Autodesk Inventor part; units mm, degrees
ref_plane "YZ Plane" through (0, 0, 0) normal (1, 0, 0) x (0, 1, 0)
ref_plane "XZ Plane" through (0, 0, 0) normal (0, 1, 0) x (-1, 0, 0)
ref_plane "XY Plane" through (0, 0, 0) normal (0, 0, 1) x (1, 0, 0)
sketch "Sketch1" plane through (0, 0, 0) normal (0, 1, 0) x (-1, 0, 0)
  line L0 (-50, 86.6025) -> (-100, 0)
  line L1 (-100, 0) -> (-50, -86.6025)
  line L2 (-50, -86.6025) -> (50, -86.6025)
  line L3 (50, -86.6025) -> (100, 0)
  line L4 (100, 0) -> (50, 86.6025)
  line L5 (50, 86.6025) -> (-50, 86.6025)
  circle A0 centre (20, -80.1075) radius 1.6
  circle A1 centre (-20, -80.1075) radius 1.6
  line L6 (-80, 0) -> (-40, 69.282)
  line L7 (-40, 69.282) -> (-20, 69.282)
  line L8 (-80, 0) -> (-40, -69.282)
  line L9 (-40, -69.282) -> (-20, -69.282)
  line L10 (20, -69.282) -> (40, -69.282)
  line L11 (40, -69.282) -> (80, 0)
  line L12 (80, 0) -> (40, 69.282)
  line L13 (40, 69.282) -> (20, 69.282)
  line L14 (-20, 69.282) -> (-20, 34.641)
  line L15 (20, 69.282) -> (20, 34.641)
  line L16 (20, -69.282) -> (20, -34.641)
  line L17 (-20, -69.282) -> (-20, -34.641)
  line L18 (-20, -34.641) -> (-40, 0)
  line L19 (-40, 0) -> (-20, 34.641)
  line L20 (20, 34.641) -> (40, 0)
  line L21 (40, 0) -> (20, -34.641)
  circle A2 centre (-10, -51.9615) radius 6.25
  circle A3 centre (10, -51.9615) radius 6.25
  circle A4 centre (-10.5, 51.9615) radius 1.65
  circle A5 centre (10.5, 51.9615) radius 1.6
  circle A6 centre (-59.3781, 57.3685) radius 1.6
  circle A7 centre (-81.8748, -18.4029) radius 1.6
  circle A8 centre (59.3781, 57.3685) radius 1.6
  circle A9 centre (81.8767, -18.3996) radius 1.6
  circle A10 centre (-30, -80.1075) radius 3
  circle A11 centre (30, -80.1075) radius 3
  dimension "d12" = 6
  dimension "d13" = 6
extrude "Extrusion1" add sketch "Sketch1" along normal blind 3
sketch "Sketch6" plane through (0, 3, 0) normal (0, 1, 0) x (1, 0, 0)
  line L0 (0, 0) -> (0, -34.641)
  line L1 (0, 0) -> (-40, 0)
  line L2 (17.5, -17.5) -> (-17.5, -17.5) construction
  line L3 (-17.5, -17.5) -> (-17.5, 17.5) construction
  line L4 (-17.5, 17.5) -> (17.5, 17.5) construction
  line L5 (17.5, 17.5) -> (17.5, -17.5) construction
  dimension "d58" = 35
  dimension "d70" = 17.5
  dimension "d72" = 17.5
decal "Decal1"
properties part number "Top Plate" material "Polycarbonate, Clear"
Can you work these out from the model? Positions are in its coordinate system, mm. A direction names the side the tool comes from. Coordinates: 2 decimals unless noted, no trailing zeros. Loops run counter-clockwise (first coordinate to the right, second up) from the corner with the lowest first, then second, coordinate; pieces in that order, holes last.
Item 1: I'm going to push flat-ended pins straight in: pin 1 (1.5 mm diameter, centred on y = 2, z = 13, fed in from +X); pin 2 (0.9 mm diameter, centred on y = 1.5, z = 50.5, fed in from -X). Where does each tip first touch, or does it pass through?
Answers below:
pin 1: stops at x = 92.93
pin 2: stops at x = -71.1
Item 2: Which directions (+Z, -Z, +X, -X, +Y, -Y) give clear straight access to the entire face, cutting with the end or side of a thin tool? Please do faces 1 (the face through (74.65, 1.48, 43.91)), 2 (the face through (60.28, 1.48, -34.16)).
Answers below:
face 1: +Z, +X, +Y, -Y
face 2: +Y, -Y
Item 3: Suppose I cut it at B-B (z = 9.5). Please give me the cut outline in (x, y), then the cut area to 3 significant figures.
Answers below:
outline: (-94.52, 0) - (-74.52, 0) - (-74.52, 3) - (-94.52, 3) - close; (-34.52, 0) - (34.52, 0) - (34.52, 3) - (-34.52, 3) - close; (74.52, 0) - (94.52, 0) - (94.52, 3) - (74.52, 3) - close
area: 327 mm2
Item 4: Suppose I cut it at C-C (y = 1.9). State how many separate pieces and enclosed holes the cut face has, then the cut area to 3 significant figures.
Answers below:
separate pieces: 1
enclosed holes: 14
area: 15,900 mm2
Item 5: If we mould it in two halves opening along X, with no side actions, what happens to faces 3 (the face through (-74.65, 1.48, -43.91)), 4 (the face through (30.14, 1.48, 17.08)), 5 (the face through (1, 3, 1)), 6 (the face through (75.35, 1.479, -42.695))? For each: released by +X, released by -X, zero draft, split by the parting line, or undercut.
Answers below:
face 3: released by -X
face 4: undercut
face 5: zero draft
face 6: released by +X
Item 6: Suppose I cut it at A-A (x = 45.5). Please give me the cut outline in (y, z), then the cut area to 3 significant figures.
Answers below:
outline: (0, -86.6) - (3, -86.6) - (3, -59.76) - (0, -59.76) - close; (0, 59.76) - (3, 59.76) - (3, 86.6) - (0, 86.6) - close
area: 161 mm2
Item 7: Please list where these lines run through material, in increasing order: L1, parallel to X at y = 1.4, z = -50.5; L2, parallel to X at y = 2.7, z = 2.5; L3, parallel to X at y = 2.5, z = -57.5.
Answers below:
L1: x = -70.84 to -50.84, -20 to -16.08, -3.92 to 3.92, 16.08 to 20, 50.84 to 70.84
L2: x = -98.56 to -78.56, -38.56 to 38.56, 78.56 to 98.56
L3: x = -66.8 to -46.8, -20 to -12.9, -7.1 to 7.1, 12.9 to 20, 46.8 to 66.8
Item 8: Suppose I cut it at D-D (x = -30). Please give me the cut outline in (y, z).
Answers below:
outline: (0, -86.6) - (3, -86.6) - (3, -83.11) - (0, -83.11) - close; (0, -77.11) - (3, -77.11) - (3, -69.28) - (0, -69.28) - close; (0, -17.32) - (3, -17.32) - (3, 17.32) - (0, 17.32) - close; (0, 69.28) - (3, 69.28) - (3, 86.6) - (0, 86.6) - close
